from build123d import *

# Parameters (mm, degrees)
SKETCH1_W                    = 130
SKETCH1_H                    = 30
SKETCH1_R                    = 2
BASE_FLANGE1_DEPTH           = 0.7366
EDGE_FLANGE1_STRIP_W         = 4.4196
EDGE_FLANGE1_STRIP_H         = 0.7366
EDGE_FLANGE1_STRIP_CUT_DEPTH = 130
EDGE_FLANGE1_DEPTH           = 130
SKETCH9_R                    = 2.05
CUT_EXTRUDE1_DEPTH           = 245.182063336


# Sheet-metal steps are written as plain solids
with BuildPart() as part:
    # Sketch1 → Base-Flange1 (new body)
    with BuildSketch(Plane(origin=(0, 0, 0), x_dir=(1, 0, 0), z_dir=(0, 1, 0))):
        Rectangle(SKETCH1_W, SKETCH1_H)
        with Locations(Location((0, -5, 0), (0, 0, 270))):
            Circle(SKETCH1_R, mode=Mode.SUBTRACT)
        with Locations(Location((-21.666666667, 5, 0), (0, 0, 270))):
            Circle(SKETCH1_R, mode=Mode.SUBTRACT)
        with Locations(Location((-43.333333333, -5, 0), (0, 0, 270))):
            Circle(SKETCH1_R, mode=Mode.SUBTRACT)
        with Locations(Location((52.33, -5, 0), (0, 0, 270))):
            Circle(SKETCH1_R, mode=Mode.SUBTRACT)
        with Locations(Location((21.67, 5, 0), (0, 0, 270))):
            Circle(SKETCH1_R, mode=Mode.SUBTRACT)
    extrude(amount=-BASE_FLANGE1_DEPTH)

    # Edge-Flange1 strip (across the edge) → Edge-Flange1 strip cut (cut)
    with BuildSketch(Plane(origin=(65, 0, -15), x_dir=(0, 0, 1), z_dir=(-1, 0, 0))):
        with Locations((-1.4732, -0.3683)):
            Rectangle(EDGE_FLANGE1_STRIP_W, EDGE_FLANGE1_STRIP_H)
    extrude(amount=EDGE_FLANGE1_STRIP_CUT_DEPTH, mode=Mode.SUBTRACT)

    # Edge-Flange1 section (across the edge) → Edge-Flange1 (add)
    with BuildSketch(Plane(origin=(65, 0, -15), x_dir=(0, 0, 1), z_dir=(-1, 0, 0))):
        with BuildLine():
            Line((-0.7366, 0.7366), (-0.7366, 20))
            Line((-0.7366, 20), (0, 20))
            Line((0, 20), (0, 0.7366))
            ThreePointArc((0, 0.7366), (0.215745145, 0.215745145), (0.7366, 0))
            Line((0.7366, 0), (0.7366, -0.7366))
            ThreePointArc((0.7366, -0.7366), (-0.30510971, -0.30510971), (-0.7366, 0.7366))
        make_face()
    extrude(amount=EDGE_FLANGE1_DEPTH)

    # Sketch9 → Cut-Extrude1 (cut, through all)
    with BuildSketch(Plane(origin=(-5.975935003, -11.740421973, -216.4732), x_dir=(-1, 0, 0), z_dir=(0, 0, -1))):
        with Locations(Location((-42.610472437, 21.740421973, 0), (0, 0, 270))):
            Circle(SKETCH9_R)
        with Locations(Location((-58.610472437, 21.740421973, 0), (0, 0, 270))):
            Circle(SKETCH9_R)
        with Locations(Location((22.862727563, 21.740421973, 0), (0, 0, 270))):
            Circle(SKETCH9_R)
        with Locations(Location((38.862727563, 21.740421973, 0), (0, 0, 270))):
            Circle(SKETCH9_R)
    extrude(amount=-CUT_EXTRUDE1_DEPTH, mode=Mode.SUBTRACT)


solid = part.part
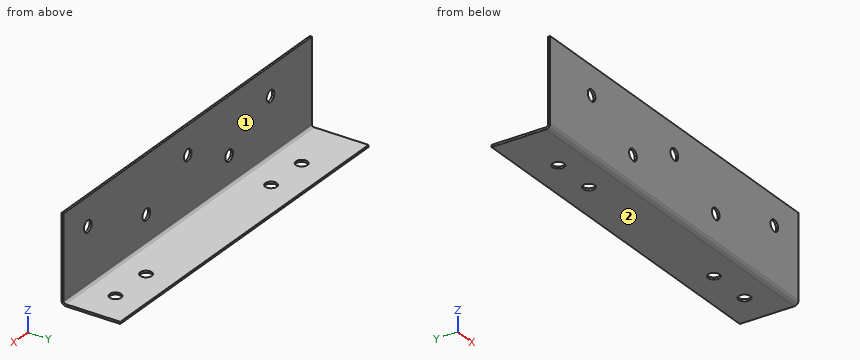
Design review of the part built by this model. Coordinates are the model's own, in mm. Face numbers are marked on the shaded views. A direction names the side the tool comes from. Give positions to 0.01 mm unless a question says otherwise; leave off trailing zeros. Loops run counter-clockwise (first coordinate to the right, second up) from the corner with the lowest first, then second, coordinate; pieces in that order, holes last. Notation, with made-up numbers: (-21, 84) -> (-9, 84) arc R37 cw to (-9, 122) -> close; hole circle Ø2 at (-16.75, 9). An arc over 180 degrees is marked (long way). One line per question, with ' | ' between items. Start each with the question number.
(1) We need section A-A (z = -5). State the section outline as (x, y) points.
(2) We need section C-C (x = 0). State the section outline as (y, z) points.
(3) For line 1 (X direction, y = -0.5, z = 5); line 2 (X direction, y = 10, z = -15.2); line 3 (Z direction, x = 29, y = 1.25), list the stretches that pass through material, from the lowest coordinate up.
(4) Insertion check: P1, Ø9.5, axis at x = -22.5, y = 9, coming from the +Z side; P2, Ø5, axis at x = 21.67, z = -5, coming from the +Y side. Each pin has a flat end and moves straight along its axis. Give the tip position at first contact, or say it passes through.
(5) For the marked faces 1 and 2, list the 3-axis set-ups (+Z, -Z, +X, -X, +Y, -Y) from which the entire face can be reached by the end or side of a thin tool; tool diameter is ignored.
(6) We need section D-D (y = 10). State the section outline as (x, z) points.
(7) We need section B-B (z = 5). State the section outline as (x, y) points.
The answers:
1) outline: (-65, -0.74) -> (-23.67, -0.74) -> (-23.67, 0) -> (-65, 0) -> close; (-19.67, -0.74) -> (19.67, -0.74) -> (19.67, 0) -> (-19.67, 0) -> close; (23.67, -0.74) -> (65, -0.74) -> (65, 0) -> (23.67, 0) -> close
2) outline: (-0.74, -14.26) arc R1.47 ccw to (0.74, -15.74) -> (20, -15.74) -> (20, -15) -> (0.74, -15) arc R0.74 cw to (0, -14.26) -> (0, 3) -> (-0.74, 3) -> close; (-0.74, 7) -> (0, 7) -> (0, 15) -> (-0.74, 15) -> close
3) line 1: x = -65 to -45.33, -41.33 to -2, 2 to 50.33, 54.33 to 65 | line 2: x = -65 to -46.89, -42.79 to -30.89, -26.79 to 34.58, 38.68 to 50.58, 54.68 to 65 | line 3: z = -15.74 to -15
4) P1: stops at z = -15 | P2: stops at y = 0
5) face 1: +Z, +X, -X, +Y | face 2: -Z, +X, -X, +Y, -Y
6) outline: (-65, -15.74) -> (-46.89, -15.74) -> (-46.89, -15) -> (-65, -15) -> close; (-42.79, -15.74) -> (-30.89, -15.74) -> (-30.89, -15) -> (-42.79, -15) -> close; (-26.79, -15.74) -> (34.58, -15.74) -> (34.58, -15) -> (-26.79, -15) -> close; (38.68, -15.74) -> (50.58, -15.74) -> (50.58, -15) -> (38.68, -15) -> close; (54.68, -15.74) -> (65, -15.74) -> (65, -15) -> (54.68, -15) -> close
7) outline: (-65, -0.74) -> (-45.33, -0.74) -> (-45.33, 0) -> (-65, 0) -> close; (-41.33, -0.74) -> (-2, -0.74) -> (-2, 0) -> (-41.33, 0) -> close; (2, -0.74) -> (50.33, -0.74) -> (50.33, 0) -> (2, 0) -> close; (54.33, -0.74) -> (65, -0.74) -> (65, 0) -> (54.33, 0) -> close
